from build123d import *

# Parameters (mm, degrees)
RESSALTO_EXTRUS_O1_DEPTH = 3


with BuildPart() as part:
    # Esboço1 → Ressalto-extrusão1 (new body)
    with BuildSketch(Plane(origin=(0, 0, 0), x_dir=(0, 0, -1), z_dir=(1, 0, 0))):
        Polygon((49, 1.499999999), (41, 1.499999999), (41, -1.500000001), (33.485947172, -1.500000001), (1.5, -1.500000001), (1.5, -6.500000001), (2.875, -6.500000001), (2.875, -9.000000001), (1.5, -9.000000001), (1.5, -14.500000001), (-1.5, -14.500000001), (-1.5, -9.000000001), (-2.875, -9.000000001), (-2.875, -6.500000001), (-1.5, -6.500000001), (-1.5, -1.500000001), (-40.999999999, -1.500000001), (-40.999999999, 1.499999999), (-48.999999999, 1.499999999), (-48.999999999, -1.500000001), (-48.999999999, -46.500000001), (-48.999999999, -49.500000001), (-40.999999999, -49.500000001), (-40.999999999, -46.500000001), (-1.5, -46.500000001), (-1.5, -41.500000001), (-2.875, -41.500000001), (-2.875, -39.000000001), (-1.5, -39.000000001), (-1.5, -33.500000001), (1.5, -33.500000001), (1.5, -39.000000001), (2.875, -39.000000001), (2.875, -41.500000001), (1.5, -41.500000001), (1.5, -46.500000001), (33.485947172, -46.500000001), (41, -46.500000001), (41, -49.5), (49, -49.5), (49, -46.500000001), (49, -24.000000001), (49, -1.500000001), align=None)
        with BuildLine():
            Line((-40.999999999, -10.109163073), (-40.999999999, -37.890836928))
            ThreePointArc((-40.999999999, -37.890836928), (-40.366648114, -38.821196622), (-39.26886168, -38.573066184))
            Line((-39.26886168, -38.573066184), (-25.670652093, -24.000000001))
            Line((-25.670652093, -24.000000001), (-39.26886168, -9.426933817))
            ThreePointArc((-39.26886168, -9.426933817), (-40.366648114, -9.17880338), (-40.999999999, -10.109163073))
        make_face(mode=Mode.SUBTRACT)
        with BuildLine():
            Line((-37.699164149, -41.500000001), (-11.642140036, -41.500000001))
            ThreePointArc((-11.642140036, -41.500000001), (-10.725017019, -40.898604281), (-10.911001717, -39.817770745))
            Line((-10.911001717, -39.817770745), (-24.670652093, -25.071690071))
            Line((-24.670652093, -25.071690071), (-38.430302469, -39.817770745))
            ThreePointArc((-38.430302469, -39.817770745), (-38.616287166, -40.898604281), (-37.699164149, -41.500000001))
        make_face(mode=Mode.SUBTRACT)
        with BuildLine():
            Line((-8.341304186, -37.890836928), (-8.341304186, -10.109163073))
            ThreePointArc((-8.341304186, -10.109163073), (-8.974656071, -9.17880338), (-10.072442506, -9.426933817))
            Line((-10.072442506, -9.426933817), (-23.670652093, -24.000000001))
            Line((-23.670652093, -24.000000001), (-10.072442506, -38.573066184))
            ThreePointArc((-10.072442506, -38.573066184), (-8.974656071, -38.821196622), (-8.341304186, -37.890836928))
        make_face(mode=Mode.SUBTRACT)
        with BuildLine():
            Line((-11.642140036, -6.500000001), (-37.699164149, -6.500000001))
            ThreePointArc((-37.699164149, -6.500000001), (-38.616287166, -7.101395721), (-38.430302469, -8.182229257))
            Line((-38.430302469, -8.182229257), (-24.670652093, -22.928309931))
            Line((-24.670652093, -22.928309931), (-10.911001717, -8.182229257))
            ThreePointArc((-10.911001717, -8.182229257), (-10.725017019, -7.101395721), (-11.642140036, -6.500000001))
        make_face(mode=Mode.SUBTRACT)
        with BuildLine():
            Line((10.911001717, -8.182229257), (24.670652093, -22.928309931))
            Line((24.670652093, -22.928309931), (38.430302469, -8.182229257))
            ThreePointArc((38.430302469, -8.182229257), (38.616287166, -7.101395721), (37.699164149, -6.500000001))
            Line((37.699164149, -6.500000001), (11.642140036, -6.500000001))
            ThreePointArc((11.642140036, -6.500000001), (10.725017019, -7.101395721), (10.911001717, -8.182229257))
        make_face(mode=Mode.SUBTRACT)
        with BuildLine():
            Line((10.072442506, -9.426933817), (23.670652093, -24.000000001))
            Line((23.670652093, -24.000000001), (10.072442506, -38.573066184))
            ThreePointArc((10.072442506, -38.573066184), (8.974656071, -38.821196622), (8.341304186, -37.890836928))
            Line((8.341304186, -37.890836928), (8.341304186, -10.109163073))
            ThreePointArc((8.341304186, -10.109163073), (8.974656071, -9.17880338), (10.072442506, -9.426933817))
        make_face(mode=Mode.SUBTRACT)
        with BuildLine():
            Line((25.670652093, -24.000000001), (39.26886168, -9.426933817))
            ThreePointArc((39.26886168, -9.426933817), (40.366648114, -9.17880338), (40.999999999, -10.109163073))
            Line((40.999999999, -10.109163073), (40.999999999, -37.890836928))
            ThreePointArc((40.999999999, -37.890836928), (40.366648114, -38.821196622), (39.26886168, -38.573066184))
            Line((39.26886168, -38.573066184), (25.670652093, -24.000000001))
        make_face(mode=Mode.SUBTRACT)
        with BuildLine():
            Line((24.670652093, -25.071690071), (10.911001717, -39.817770745))
            ThreePointArc((10.911001717, -39.817770745), (10.725017019, -40.898604281), (11.642140036, -41.500000001))
            Line((11.642140036, -41.500000001), (37.699164149, -41.500000001))
            ThreePointArc((37.699164149, -41.500000001), (38.616287166, -40.898604281), (38.430302469, -39.817770745))
            Line((38.430302469, -39.817770745), (24.670652093, -25.071690071))
        make_face(mode=Mode.SUBTRACT)
    extrude(amount=RESSALTO_EXTRUS_O1_DEPTH)


solid = part.part
Source: CAD feature listing. Evaluate the final solid. Frame: model axes, mm. A direction names the side the tool comes from. Give positions to 0.01 mm unless a question says otherwise; leave off trailing zeros. Write each loop counter-clockwise with the first axis right and the second up, starting at its lowest first coordinate (ties: lowest second). Pieces come first, ordered by that corner, then holes. Notation, with made-up numbers: (87.5, 16) -> (94.5, 16) arc R18 cw to (94.5, 24) -> close; hole circle Ø4 at (-34, 75.5). An arc over 180 degrees is marked (long way). Return JSON: item names as keys, results as strings. Group by question number.
1. Section B-B, the plane z = 16.5. Output: boundary loops of the cut face in (x, y), then the cut area to 3 significant figures.
2. Section A-A, the plane y = -42.5. Output: boundary loops of the cut face in (x, z), then the cut area to 3 significant figures.
3. Section D-D, the plane x = 1.25. Count the separate pieces of the cut face and the enclosed holes in it, then the cut area to 3 significant figures.
4. Pin query (flat end, axial travel): pin 1 Ø1 at (x, z) = (0.5, -9) entering from +Y; pin 2 Ø0.9 at (x, z) = (2, -21) entering from -Y; pin 3 Ø0.9 at (x, z) = (2, -0.5) entering from -Y. Return the tip coordinate at first contact, or that it passes through.
5. Mould query, pull axis Z, two halves, no side actions, for faces 4 (the face through (3, -24, 0)), 5 (the face through (1.48, -7.09, -10.73)), 6 (the face through (1, 0, -41)), 7 (the face through (1, -24, 49)). Classes: +Z half, -Z half, draft (parallel to the pull), parting line (faces both ways), or undercut.
6. Access query for faces 1 (the face through (1, -40, 2.875)), 2 (the face through (1, -36, -1.5)), 3 (the face through (1, -12, 1.5)). Directions: +Z, -Z, +X, -X, +Y, -Y. A direction counts if a zero-diameter tool reaches every point of the face in a straight line with its end or side. Return the directions, or none.
7. Section C-C, the plane y = -21. Output: boundary loops of the cut face in (x, z).
8. Material intervals for line 1 (Y direction, x = 2.65, z = 13); line 2 (Y direction, x = 2.05, z = 12.5); line 3 (Z direction, x = 0.45, y = -4), sorted ascending. Write a range as from..to.
Determined:
{
 "1": {"outline": "(0, -46.5) -> (3, -46.5) -> (3, -41.5) -> (0, -41.5) -> close; (0, -33.83) -> (3, -33.83) -> (3, -31.68) -> (0, -31.68) -> close; (0, -16.32) -> (3, -16.32) -> (3, -14.17) -> (0, -14.17) -> close; (0, -6.5) -> (3, -6.5) -> (3, -1.5) -> (0, -1.5) -> close", "area": "42.9 mm2"},
 "2": {"outline": "(0, -49) -> (3, -49) -> (3, -1.5) -> (0, -1.5) -> close; (0, 1.5) -> (3, 1.5) -> (3, 49) -> (0, 49) -> close", "area": "285 mm2"},
 "3": {"separate pieces": "1", "enclosed holes": "8", "area": "2,420 mm2"},
 "4": {"pin 1": "stops at y = -1.5", "pin 2": "stops at y = -46.5", "pin 3": "stops at y = -33.5"},
 "5": {"face 4": "draft", "face 5": "undercut", "face 6": "undercut", "face 7": "+Z half"},
 "6": {"face 1": "+X, -X", "face 2": "+X, -X, -Y", "face 3": "+X, -X, +Y"},
 "7": {"outline": "(0, -49) -> (3, -49) -> (3, -41) -> (0, -41) -> close; (0, -28.47) -> (3, -28.47) -> (3, -26.47) -> (0, -26.47) -> close; (0, -22.87) -> (3, -22.87) -> (3, -20.87) -> (0, -20.87) -> close; (0, -8.34) -> (3, -8.34) -> (3, 8.34) -> (0, 8.34) -> close; (0, 20.87) -> (3, 20.87) -> (3, 22.87) -> (0, 22.87) -> close; (0, 26.47) -> (3, 26.47) -> (3, 28.47) -> (0, 28.47) -> close; (0, 41) -> (3, 41) -> (3, 49) -> (0, 49) -> close"},
 "8": {"line 1": "y = -46.5..-41.5, -37.58..-35.44, -12.56..-10.42, -6.5..-1.5", "line 2": "y = -46.5..-41.5, -38.11..-35.97, -12.03..-9.89, -6.5..-1.5", "line 3": "z = -49..-1.5, 1.5..49"}
}
